Could you check a few things on this drawing? It's one solid part, dimensions in mm from its lowest x, y, z. A direction names the side the tool comes from. Give positions to 0.01 mm unless a question says otherwise; leave off trailing zeros. Order: outer loops, then holes, each group sorted by start corner. A loop starts at its lowest first (then second) coordinate and runs counter-clockwise, first axis right, second up.
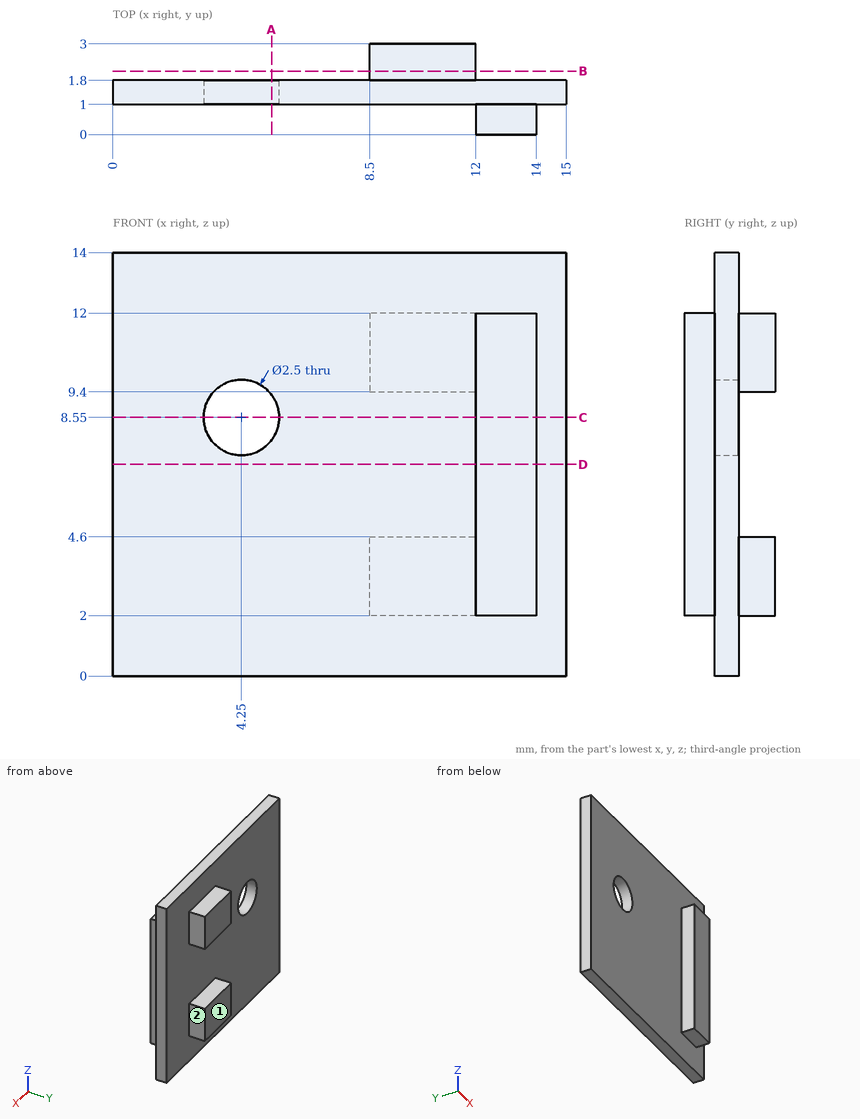
Item 1: Imagine slicing it at A-A on x = 5.25. List the corners of the cut face in (y, z) for me, then the cut area to 3 significant figures.
Findings:
outline: (1, 0) - (1.8, 0) - (1.8, 7.8) - (1, 7.8) - close; (1, 9.3) - (1.8, 9.3) - (1.8, 14) - (1, 14) - close
area: 10.0 mm2
Item 2: Imagine slicing it at B-B on y = 2.1. List the corners of the cut face in (x, z) for me, then the cut area to 3 significant figures.
Findings:
outline: (8.5, 2) - (12, 2) - (12, 4.6) - (8.5, 4.6) - close; (8.5, 9.4) - (12, 9.4) - (12, 12) - (8.5, 12) - close
area: 18.2 mm2
Item 3: Imagine slicing it at D-D on z = 7. List the corners of the cut face in (x, y) for me, then the cut area to 3 significant figures.
Findings:
outline: (0, 1) - (12, 1) - (12, 0) - (14, 0) - (14, 1) - (15, 1) - (15, 1.8) - (0, 1.8) - close
area: 14.0 mm2
Item 4: Imagine slicing it at C-C on z = 8.55. List the corners of the cut face in (x, y) for me, then the cut area to 3 significant figures.
Findings:
outline: (0, 1) - (3, 1) - (3, 1.8) - (0, 1.8) - close; (5.5, 1) - (12, 1) - (12, 0) - (14, 0) - (14, 1) - (15, 1) - (15, 1.8) - (5.5, 1.8) - close
area: 12.0 mm2
Item 5: Please list where these lines run through material, in increasing order: line 1 along X through (y, z) = (1.45, 8.55); line 2 along Z through (x, y) = (4.25, 1.3); line 3 along Z through (x, y) = (9.5, 2.3).
Findings:
line 1: x = 0 to 3, 5.5 to 15
line 2: z = 0 to 7.3, 9.8 to 14
line 3: z = 2 to 4.6, 9.4 to 12
Item 6: For pin 1 (1.3 mm diameter, centred on y = 2.5, z = 10.5, fed in from +X); pin 2 (1 mm diameter, centred on x = 11, y = 2.5, fed in from -Z); pin 3 (3 mm diameter, centred on x = 4.25, z = 8.55, fed in from -Y), each with a flat end and sliding along its axis, tell me the tip position at first contact or that it passes through.
Findings:
pin 1: stops at x = 12
pin 2: stops at z = 2
pin 3: stops at y = 1
Item 7: For the marked faces 1 and 2, which set-ups out of +Z, -Z, +X, -X, +Y, -Y let a thin tool reach every point of the face, with its end or its side?
Findings:
face 1: +Z, -Z, +X, -X, +Y
face 2: +Z, -Z, +X, +Y
